Can you work these out from the model? Positions are in its coordinate system, mm. A direction names the side the tool comes from. Round coordinates to 2 decimals unless told otherwise and drop trailing zeros. Write each loop counter-clockwise with the first axis right and the second up, starting at its lowest first coordinate (ties: lowest second). Pieces come first, ordered by that corner, then holes. Notation, with made-up numbers: M -38.5,14.5 L -30.5,14.5 A26 ccw -30.5,47.5 Z; hole C 30,-32 d9. An arc over 180 degrees is marked long. Answer as a JSON object with one key per item and string values. Group by question number.
1) Suppose I cut it at A-A, the plane y = 0. Write out the boundary of the cut face in (x, z).
2) Please list where these lines run through material, in increasing order: L1, parallel to Z at x = 22.5, y = -17; L2, parallel to X at y = 7.5, z = 7; L3, parallel to X at y = -4, z = -2. Write a range as [from, to].
3) I'm going to push a flat-ended pin straight in: pin 1 Ø1.5 at (x, y) = (15, -10.5) entering from -Z. Where does the tip first touch, or does it pass through?
4) Suppose I cut it at B-B, the plane x = 0. Write out the boundary of the cut face in (y, z).
5) Suppose I cut it at C-C, the plane z = -26.5. Write out the boundary of the cut face in (x, y), and give its area (3 significant figures).
6) Suppose I cut it at D-D, the plane x = -24.5. Write out the boundary of the cut face in (y, z), and give its area (3 significant figures).
7) On a 3-axis mill with a long thin cutter (end or side, diameter ignored), from which of +Z, -Z, +X, -X, +Y, -Y can I reach the whole of each face in a straight line? I mean faces 1 (the flat face through (6, 9, -20)), 2 (the flat face through (0, 0, -45)). Say none if no direction works.
from build123d import *

# Parameters (mm, degrees)
F1_DEPTH = 20
F2_R     = 10
F3_DEPTH = 25


with BuildPart() as f1:
    # F0 (on Top) → F1 (new body, symmetric)
    with BuildSketch(Plane.XY):
        with BuildLine():
            Line((22.36068, 20), (-22.36068, 20))
            ThreePointArc((-22.36068, 20), (-30, 0), (-22.36068, -20))
            Line((-22.36068, -20), (22.36068, -20))
            ThreePointArc((22.36068, -20), (30, 0), (22.36068, 20))
        make_face()
    extrude(amount=F1_DEPTH, both=True)

    # F2 (on face) → F3 (join)
    with BuildSketch(Plane(origin=(0, 0, -20), x_dir=(1, 0, 0), z_dir=(0, 0, -1))):
        Circle(F2_R)
    extrude(amount=F3_DEPTH)


solid = f1.part
Results:
{
 "1": {"outline": "M -30,-20 L -10,-20 L -10,-45 L 10,-45 L 10,-20 L 30,-20 L 30,20 L -30,20 Z"},
 "2": {"L1": "[-20, 20]", "L2": "[-29.05, 29.05]", "L3": "[-29.73, 29.73]"},
 "3": {"pin 1": "z = -20"},
 "4": {"outline": "M -20,-20 L -10,-20 L -10,-45 L 10,-45 L 10,-20 L 20,-20 L 20,20 L -20,20 Z"},
 "5": {"outline": "C 0,0 d20", "area": "314 mm^2"},
 "6": {"outline": "M -17.31,-20 L 17.31,-20 L 17.31,20 L -17.31,20 Z", "area": "1,390 mm^2"},
 "7": {"face 1": "-Z", "face 2": "-Z, +X, -X, +Y, -Y"}
}
